Verification items for the finished model (mm, model axes). A direction names the side the tool comes from. Coordinates: 2 decimals unless noted, no trailing zeros. Loops run counter-clockwise (first coordinate to the right, second up) from the corner with the lowest first, then second, coordinate; pieces in that order, holes last. Notation, with made-up numbers: (78, -12.5) - (109, -12.5) arc R23 ccw to (109, 17.5) - close; hole circle Ø2 at (84.25, 34). An arc over 180 degrees is marked (long way). One line per item, written item: value. Start each with the question number.
(1) Section check C-C (z = 1.45). Record the boundary of the cut face in (x, y) (3 decimals).
(2) Gauge pin test, flat ends, axial feed: P1, Ø6, axis at x = 3, y = 6.5, coming from the +Z side; P2, Ø1, axis at y = -7, z = 1, coming from the +X side. Record the tip position at first contact, or that the pin passes through.
(3) Thickness scan on probe 1 along Z at (x, y) = (7.75, 6); probe 2 along Z at (x, y) = (6.25, 3); probe 3 along Y at (x, z) = (8.25, 0.45). Record the ranges inside material, lowest first. Write a range as [from, to].
(4) Section check D-D (z = 4). Record the boundary of the cut face in (x, y) (3 decimals).
(5) Section check A-A (x = 0). Record the boundary of the cut face in (y, z) (3 decimals).
(6) Set-up check for faces 1 (the face through (0, 0, 4.5)), 2 (the face through (0, 9, 1)): record each of +Z, -Z, +X, -X, +Y, -Y from which the full face is reachable in a straight line by a thin tool's end or side.
```python
from build123d import *

# Parameters (mm, degrees)
F0_R     = 10.5
F1_DEPTH = 1
F2_R     = 3.925
F3_DEPTH = 3.5
F4_SIZE  = 0.75
F5_R     = 0.5
F6_R     = 8.536956
F7_DEPTH = 0.2


with BuildPart() as f1:
    # F0 (on Top) → F1 (new body)
    with BuildSketch(Plane.XY):
        Circle(F0_R)
    extrude(amount=F1_DEPTH)

    # F2 (on face) → F3 (join)
    with BuildSketch(Plane.XY.offset(1)):
        Circle(F2_R)
    extrude(amount=F3_DEPTH)

    # F4
    f4_edges = [f1.edges().sort_by_distance(p)[0] for p in [
        (-3.925, 0, 4.5),
    ]]
    chamfer(f4_edges, length=F4_SIZE)

    # F5
    f5_edges = [f1.edges().sort_by_distance(p)[0] for p in [
        (-10.5, 0, 0),
    ]]
    fillet(f5_edges, radius=F5_R)

    # F6 (on face) → F7 (join)
    with BuildSketch(Plane.XY.offset(1)):
        Circle(F6_R)
    extrude(amount=F7_DEPTH)


solid = f1.part
```
Responses:
1. outline: circle Ø7.85 at (0, 0)
2. P1: stops at z = 1.2
2. P2: stops at x = 8.25
3. probe 1: z = [0, 1]
3. probe 2: z = [0, 1.2]
3. probe 3: y = [-6.49, 6.49]
4. outline: circle Ø7.35 at (0, 0)
5. outline: (-10.5, 0.5) arc R0.5 ccw to (-10, 0) - (10, 0) arc R0.5 ccw to (10.5, 0.5) - (10.5, 1) - (8.537, 1) - (8.537, 1.2) - (3.925, 1.2) - (3.925, 3.75) - (3.175, 4.5) - (-3.175, 4.5) - (-3.925, 3.75) - (-3.925, 1.2) - (-8.537, 1.2) - (-8.537, 1) - (-10.5, 1) - close
6. face 1: +Z, +X, -X, +Y, -Y
6. face 2: +Z
